```python
from build123d import *

# Parameters (mm, degrees)
F0_W     = 12.7
F0_H     = 3.175
F0_W_2   = 6.35
F0_H_2   = 12.7
F1_DEPTH = 3.175
F2_DEPTH = 9.525
F3_R     = 0.79375


with BuildPart() as f1:
    # F0 (on Top) → F1 (new body)
    with BuildSketch(Plane.XY):
        Polygon((-3.175, 0), (-12.7, 0), (-12.7, -6.35), (12.7, -6.35), (12.7, 0), (3.175, 0), align=None)
        with Locations((0, -3.175)):
            Rectangle(F0_W, F0_H, mode=Mode.SUBTRACT)
        with Locations((0, -3.175)):
            Rectangle(F0_W, F0_H)
        with Locations((0, 6.35)):
            Rectangle(F0_W_2, F0_H_2)
    extrude(amount=-F1_DEPTH)

    # F0 (on Top) → F2 (join)
    with BuildSketch(Plane.XY):
        with Locations((0, -3.175)):
            Rectangle(F0_W, F0_H)
    extrude(amount=F2_DEPTH)

    # F3
    f3_edges = [f1.edges().sort_by_distance(p)[0] for p in [
        (0, -4.7625, 9.525),
        (0, -1.5875, 9.525),
        (0, -1.5875, 0),
        (0, -4.7625, 0),
    ]]
    fillet(f3_edges, radius=F3_R)


solid = f1.part
```
Here's how the part is built. I have some questions about the finished solid (model axes, mm). A direction names the side the tool comes from. Give positions to 0.01 mm unless a question says otherwise; leave off trailing zeros. Order: outer loops, then holes, each group sorted by start corner. A loop starts at its lowest first (then second) coordinate and runs counter-clockwise, first axis right, second up. Notation, with made-up numbers: (36, -18) -> (57, -18) arc R31 cw to (57, 13) -> close; hole circle Ø10 at (66.5, -0.5). An arc over 180 degrees is marked (long way). Use CSV: the item, a comma, the result in double quotes. Start each with the question number.
Item 1: If I drill on probe 1 along X at (y, z) = (-2.5, 3.75); probe 2 along Y at (x, z) = (4.5, 7); probe 3 along Y at (x, z) = (-5.25, -1), over which ranges is the centre line in solid material (lowest first)? Write a range as [from, to].
Item 2: Suppose I cut it at C-C (y = 10). List the corners of the cut face in (x, z) for me (3 decimals).
Item 3: Suppose I cut it at B-B (z = -1). List the corners of the cut face in (x, y) for me (3 decimals).
Item 4: I'm going to push flat-ended pins straight in: P1, Ø1.5, axis at x = 4, y = -0.5, coming from the +Z side; P2, Ø2.5, axis at x = -8, z = -1, coming from the +Y side; P3, Ø1.5, axis at x = -8.5, z = 2.5, coming from the +Y side; P4, Ø1.4, axis at y = -2, z = 5, coming from the +X side. Where does each tip first touch, or does it pass through?
Item 5: On a 3-axis mill with a long thin cutter (end or side, diameter ignored), from which of +Z, -Z, +X, -X, +Y, -Y can I reach the whole of each face in a straight line? I mean faces 1 (the flat face through (3.175, 6, -2)), 2 (the flat face through (6.35, -3, 5)), 3 (the flat face through (-6.35, -3, 5)), 4 (the flat face through (-3.175, 6, -2)). Say none if no direction works.
Item 6: Suppose I cut it at D-D (x = 9.25). List the corners of the cut face in (y, z) for me (3 decimals).
Answer block:
1,probe 1,"x = [-6.35, 6.35]"
1,probe 2,"y = [-4.76, -1.59]"
1,probe 3,"y = [-6.35, 0]"
2,outline,"(-3.175, -3.175) -> (3.175, -3.175) -> (3.175, 0) -> (-3.175, 0) -> close"
3,outline,"(-12.7, -6.35) -> (12.7, -6.35) -> (12.7, 0) -> (3.175, 0) -> (3.175, 12.7) -> (-3.175, 12.7) -> (-3.175, 0) -> (-12.7, 0) -> close"
4,P1,"stops at z = 0.14"
4,P2,"stops at y = 0"
4,P3,"passes through"
4,P4,"stops at x = 6.35"
5,face 1,"+Z, -Z, +X, +Y"
5,face 2,"+Z, +X, +Y, -Y"
5,face 3,"+Z, -X, +Y, -Y"
5,face 4,"+Z, -Z, -X, +Y"
6,outline,"(-6.35, -3.175) -> (0, -3.175) -> (0, 0) -> (-6.35, 0) -> close"
